```python
from build123d import *

# Parameters (mm, degrees)
SKETCH1_R           = 2.1
SKETCH1_R_2         = 6
SKETCH1_R_3         = 11
SKETCH1_R_4         = 2
SKETCH1_R_5         = 1.6
BOSS_EXTRUDE1_DEPTH = 8


with BuildPart() as part:
    # Sketch1 → Boss-Extrude1 (new body)
    with BuildSketch(Plane.XY):
        with BuildLine():
            Line((-58.634566509, -94.315974521), (11.365433491, -94.315974521))
            ThreePointArc((11.365433491, -94.315974521), (14.900967397, -92.851508427), (16.365433491, -89.315974521))
            Line((16.365433491, -89.315974521), (16.365433491, -55.206132823))
            ThreePointArc((16.365433491, -55.206132823), (18.877822606, -43.188177597), (25.994183345, -33.18314103))
            Line((25.994183345, -33.18314103), (78.736683637, 15.603630397))
            ThreePointArc((78.736683637, 15.603630397), (85.853044376, 25.608666964), (88.365433491, 37.62662219))
            Line((88.365433491, 37.62662219), (88.365433491, 93.348359509))
            ThreePointArc((88.365433491, 93.348359509), (82.507569115, 107.490495133), (68.365433491, 113.348359509))
            Line((68.365433491, 113.348359509), (46.365433491, 113.348359509))
            ThreePointArc((46.365433491, 113.348359509), (32.223297867, 107.490495133), (26.365433491, 93.348359509))
            Line((26.365433491, 93.348359509), (26.365433491, 66.006418518))
            ThreePointArc((26.365433491, 66.006418518), (24.005761373, 54.343988473), (17.29794852, 44.516192494))
            Line((17.29794852, 44.516192494), (-54.567081538, -25.483807506))
            ThreePointArc((-54.567081538, -25.483807506), (-61.274894391, -35.311603484), (-63.634566509, -46.97403353))
            Line((-63.634566509, -46.97403353), (-63.634566509, -89.315974521))
            ThreePointArc((-63.634566509, -89.315974521), (-62.170100415, -92.851508427), (-58.634566509, -94.315974521))
        make_face()
        with Locations((-56.634566509, -57.065974521)):
            Circle(SKETCH1_R, mode=Mode.SUBTRACT)
        with Locations((-30.634566509, -57.065974521)):
            Circle(SKETCH1_R, mode=Mode.SUBTRACT)
        with Locations((-30.634566509, -87.565974521)):
            Circle(SKETCH1_R, mode=Mode.SUBTRACT)
        with Locations((-56.634566509, -87.565974521)):
            Circle(SKETCH1_R, mode=Mode.SUBTRACT)
        with Locations((9.365433491, -87.565974521)):
            Circle(SKETCH1_R, mode=Mode.SUBTRACT)
        with Locations((-16.634566509, -87.565974521)):
            Circle(SKETCH1_R, mode=Mode.SUBTRACT)
        with Locations((-16.634566509, -57.065974521)):
            Circle(SKETCH1_R, mode=Mode.SUBTRACT)
        with Locations((9.365433491, -57.065974521)):
            Circle(SKETCH1_R, mode=Mode.SUBTRACT)
        with Locations((57.365433491, 99.348359509)):
            Circle(SKETCH1_R_2, mode=Mode.SUBTRACT)
        with Locations((57.365433491, 27.408359509)):
            Circle(SKETCH1_R_2, mode=Mode.SUBTRACT)
        with Locations((57.365433491, 63.378359509)):
            Circle(SKETCH1_R_3, mode=Mode.SUBTRACT)
        with Locations((84.365433491, 37.62662219)):
            Circle(SKETCH1_R_4, mode=Mode.SUBTRACT)
        with Locations((84.375885899, 88.528341433)):
            Circle(SKETCH1_R_4, mode=Mode.SUBTRACT)
        with Locations((47.365433491, 99.348359509)):
            Circle(SKETCH1_R_5, mode=Mode.SUBTRACT)
        with Locations((47.365433491, 27.408359509)):
            Circle(SKETCH1_R_5, mode=Mode.SUBTRACT)
        with Locations((67.365433491, 99.348359509)):
            Circle(SKETCH1_R_5, mode=Mode.SUBTRACT)
        with Locations((67.365433491, 27.408359509)):
            Circle(SKETCH1_R_5, mode=Mode.SUBTRACT)
        with Locations((84.370659695, 63.077481811)):
            Circle(SKETCH1_R_4, mode=Mode.SUBTRACT)
    extrude(amount=BOSS_EXTRUDE1_DEPTH)


solid = part.part
```
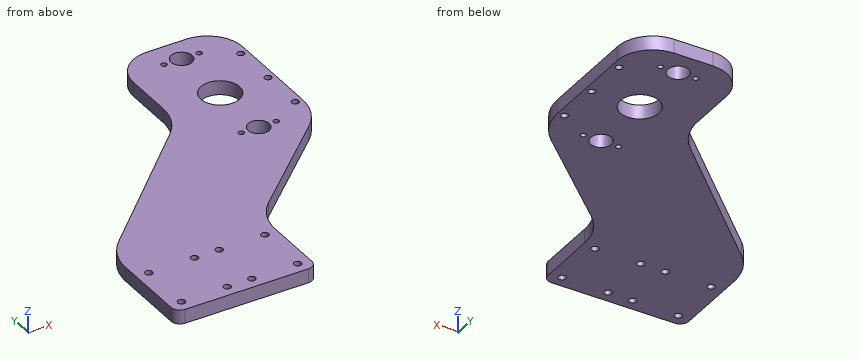
Geometry check sheet. Reference: the model listing, model coordinates, mm. Coordinates: 2 decimals unless noted, no trailing zeros. Write each loop counter-clockwise with the first axis right and the second up, starting at its lowest first coordinate (ties: lowest second). Pieces come first, ordered by that corner, then holes. Notation, with made-up numbers: M 20.25,-10.75 L 36.25,-10.75 A25 cw 36.25,5.25 Z; hole C 70,74 d8. An arc over 180 degrees is marked long. Use one line per item in the form item = value. Start each with the question number.
1) Section check B-B on z = 5.75. State how many separate pieces and enclosed holes the cut face has, and give its area (3 significant figures).
2) Section check C-C on x = 61. Enter the section's corners in (y, z), and give its area (3 significant figures).
3) Go/stop test with flat-tipped pins: pin 1 Ø1 at (x, z) = (61, 1.5) entering from -Y; pin 2 Ø2 at (x, z) = (53, 1) entering from -Y. Record where each tip stops, or that it passes through.
4) Section check A-A on y = 71. Enter the section's corners in (x, z), and give its area (3 significant figures).
5) Section check D-D on y = -70. Enter the section's corners in (x, z), and give its area (3 significant figures).
6) Thickness scan on probe 1 along Y at (x, z) = (11, 3.75); probe 2 along X at (y, z) = (86, 3.5); probe 3 along X at (y, z) = (38, 1.75). Record the ranges inside material, lowest first. Write a range as from..to.
Responses:
q1.separate_pieces = 1
q1.enclosed_holes = 18
q1.area = 15,100 mm2
q2.outline = M -0.8,0 L 22.63,0 L 22.63,8 L -0.8,8 Z; M 32.18,0 L 53,0 L 53,8 L 32.18,8 Z; M 73.76,0 L 94.57,0 L 94.57,8 L 73.76,8 Z; M 104.12,0 L 113.35,0 L 113.35,8 L 104.12,8 Z
q2.area = 594 mm2
q3.pin_1 = -1.27
q3.pin_2 = -9.13
q4.outline = M 26.37,0 L 49.43,0 L 49.43,8 L 26.37,8 Z; M 65.3,0 L 88.37,0 L 88.37,8 L 65.3,8 Z
q4.area = 369 mm2
q5.outline = M -63.63,0 L 16.37,0 L 16.37,8 L -63.63,8 Z
q5.area = 640 mm2
q6.probe_1 = -94.32..-88.88, -86.25..-58.38, -55.75..38.38
q6.probe_2 = 26.37..88.37
q6.probe_3 = 10.61..82.4, 86.33..88.37
